Geometry check sheet. Reference: the model listing, model coordinates, mm. Face numbers are marked on the shaded views. Coordinates: 2 decimals unless noted, no trailing zeros. Write each loop counter-clockwise with the first axis right and the second up, starting at its lowest first coordinate (ties: lowest second). Pieces come first, ordered by that corner, then holes. Notation, with made-up numbers: M 89.5,10.25 L 126.5,10.25 A19 cw 126.5,15.25 Z; hole C 63.5,25.25 d5. An arc over 180 degrees is marked long. Answer as a JSON object with one key per item and string values. Group by question number.
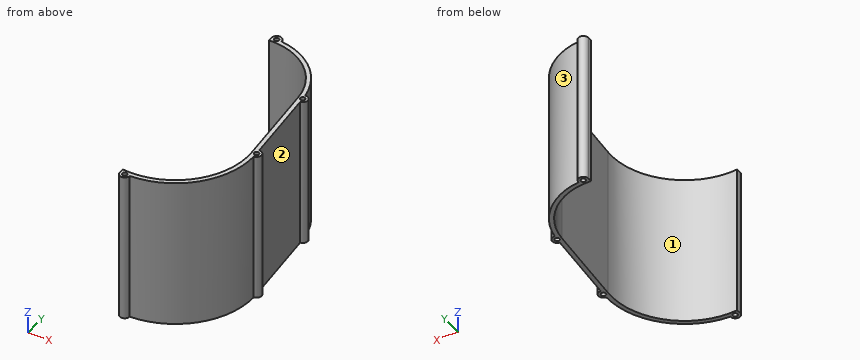
Autodesk Inventor part; units mm, degrees
ref_plane "YZ Plane" through (0, 0, 0) normal (1, 0, 0) x (0, 1, 0)
ref_plane "XZ Plane" through (0, 0, 0) normal (0, 1, 0) x (-1, 0, 0)
ref_plane "XY Plane" through (0, 0, 0) normal (0, 0, 1) x (1, 0, 0)
ref_plane "Work Plane1" through (0, 0, 0) normal (0, 0, 1) x (1, 0, 0)
sketch "Sketch1" plane through (0, 0, 0) normal (0, 0, 1) x (1, 0, 0)
  circle A0 centre (-55.8916, -14.7421) radius 1.397
  circle A1 centre (-83.8916, 18.2579) radius 1.397
  circle A2 centre (-83.8916, -14.7421) radius 1.397
  circle A3 centre (-55.8916, 18.2579) radius 1.397
  circle A4 centre (2.1895, 105.4705) radius 2.159
  circle A5 centre (-2.169, -104.4843) radius 2.159
  circle A6 centre (60.6164, 51.7463) radius 2.159
  circle A7 centre (-58.4167, 54.2173) radius 2.159
  arc A8 (6.6818, 105.2084) -> (-2.3099, 105.3951) centre (2.1895, 105.4705) ccw
  arc A9 (-2.3099, 105.3951) -> (-57.5952, 58.6417) centre (0.9442, 45.4834) ccw construction
  arc A10 (-57.5952, 58.6417) -> (-59.0718, 49.7652) centre (-58.4167, 54.2173) ccw
  line L0 (-59.0718, 49.7652) -> (-63.1925, 21.7579)
  line L1 (-87.8916, 21.7579) -> (-63.1925, 21.7579)
  line L2 (-87.8916, -18.2421) -> (-87.8916, 21.7579)
  line L3 (-87.8916, -18.2421) -> (-74.0344, -26.2425)
  arc A11 (-74.0344, -26.2425) -> (-70.4822, -28.7807) centre (-69.9706, -24.3098) ccw
  arc A12 (-70.4822, -28.7807) -> (-6.6627, -104.2463) centre (-0.7162, -34.4994) ccw construction
  arc A13 (-6.6627, -104.2463) -> (2.3307, -104.433) centre (-2.169, -104.4843) ccw
  arc A14 (2.3307, -104.433) -> (69.2271, -31.6809) centre (-0.7162, -34.4994) ccw
  arc A15 (69.2271, -31.6809) -> (68.4317, -22.7173) centre (68.9014, -27.1927) ccw
  line L4 (68.4317, -22.7173) -> (61.0862, 47.2708)
  arc A16 (61.0862, 47.2708) -> (59.9792, 56.2009) centre (60.6164, 51.7463) ccw
  arc A17 (59.9792, 56.2009) -> (6.6818, 105.2084) centre (0.9442, 45.4834) ccw
  circle A18 centre (-69.9706, -24.3098) radius 2.159
  circle A19 centre (68.9014, -27.1927) radius 2.159
  circle A20 centre (0.9442, 45.4834) radius 17.5
  circle A21 centre (-0.7162, -34.4994) radius 17.5
  circle A22 centre (-66.7556, 10.6536) radius 4
  circle A23 centre (-75.8916, -7.1378) radius 4
  line L5 (-6.6627, -104.2463) -> (-2.3099, 105.3951) construction
  line L6 (-6.6627, -104.2463) -> (-6.5797, -100.2463)
  line L7 (-2.3099, 105.3951) -> (-2.393, 101.3951)
  arc A24 (-6.5797, -100.2463) -> (64.9314, -27.6121) centre (-0.7162, -34.4994) ccw
  arc A25 (56.6497, 51.3276) -> (-2.393, 101.3951) centre (0.9442, 45.4834) ccw
  line L8 (64.9314, -27.6121) -> (56.6497, 51.3276)
  point P0 (0, 0)
  dimension "d0" = 4
  dimension "d1" = 4
extrude "Extrusion1" add sketch "Sketch1" along normal blind 135 contours A17 A16 L4 A15 A14 A13 L6 A24 L8 A25 L7 A8
properties part number "case bottom half"
1) Section check D-D (y = 81.5). Record the cut outline in (x, z).
2) Section check A-A (x = 40). Record the cut outline in (y, z), then the cut area to 3 significant figures.
3) Material ranges on probe 1 along X at (y, z) = (51.5, 35); probe 2 along Y at (x, z) = (1.5, 36); probe 3 along X at (y, z) = (9, 41.5), recorded low to high. Write a range as [from, to].
4) Section check B-B (z = 65). Record the cut outline in (x, y), then the cut area to 3 significant figures.
5) Section check C-C (x = 14.5). Record the cut outline in (y, z), then the cut area to 3 significant figures.
6) Go/stop test with flat-tipped pins: pin 1 Ø4 at (y, z) = (-8.5, 41.5) entering from +X; pin 2 Ø10 at (y, z) = (81, 120) entering from -X; pin 3 Ø5 at (y, z) = (-32, 26) entering from +X. Record where each tip stops, or that it passes through.
7) Draft check along Y on the marked faces 1, 2 and 3. Enter one of: +Y half, -Y half, draft (parallel to the pull), parting line (faces both ways), or undercut.
Entries:
{
 "1": {"outline": "M 43.84,0 L 48.93,0 L 48.93,135 L 43.84,135 Z"},
 "2": {"outline": "M -91.44,0 L -86.45,0 L -86.45,135 L -91.44,135 Z; M 85.63,0 L 91.03,0 L 91.03,135 L 85.63,135 Z", "area": "1,400 mm^2"},
 "3": {"probe 1": "[56.63, 58.47], [62.76, 65.11]", "probe 2": "[-107.09, -100.47], [101.49, 103.42], [107.52, 109.92]", "probe 3": "[61.09, 65.1]"},
 "4": {"outline": "M -6.66,-104.25 A4.5 ccw long 2.33,-104.43 A70 ccw 69.23,-31.68 A4.5 ccw long 68.43,-22.72 L 61.09,47.27 A4.5 ccw long 59.98,56.2 A60 ccw 6.68,105.21 A4.5 ccw long -2.31,105.4 L -2.39,101.4 A56.01 cw 56.65,51.33 L 64.93,-27.61 A66.01 cw -6.58,-100.25 Z; hole C -2.17,-104.48 d4.32; hole C 2.19,105.47 d4.32; hole C 60.62,51.75 d4.32; hole C 68.9,-27.19 d4.32", "area": "1,220 mm^2"},
 "5": {"outline": "M -102.83,0 L -98.73,0 L -98.73,135 L -102.83,135 Z; M 99.83,0 L 103.93,0 L 103.93,135 L 99.83,135 Z", "area": "1,110 mm^2"},
 "6": {"pin 1": "x = 67.15", "pin 2": "x = 39.62", "pin 3": "x = 72.76"},
 "7": {"face 1": "undercut", "face 2": "undercut", "face 3": "+Y half"}
}
